Check sheet for the modelled part. Datum: model origin and axes. Units: mm. A direction names the side the tool comes from. Give positions to 0.01 mm unless a question says otherwise; leave off trailing zeros. Order: outer loops, then holes, each group sorted by start corner. A loop starts at its lowest first (then second) coordinate and runs counter-clockwise, first axis right, second up.
Item 1: Sectioned sample at B-B on x = 38.5. Record the boundary of the cut face in (y, z).
Item 2: Sectioned sample at A-A on x = 20.5. Record the boundary of the cut face in (y, z).
Item 3: Access from +Z, -Z, +X, -X, +Y, -Y to the whole of each face (thin tool, end or side, straight path). Record for faces 4 (the flat face through (63.09, -1.23, 1.48)), 5 (the flat face through (22, -4.25, 2)), 6 (the cylindrical face through (-10.248, 0.225, 1.479)), 7 (the flat face through (16, -10.25, 1)), 8 (the flat face through (54, -14.25, 9)).
Item 4: Material ranges on line 1 along Z through (x, y) = (68.5, -15.65); line 2 along Z through (x, y) = (63, -4); line 3 along Y through (x, z) = (36, 11), recorded low to high.
Item 5: Sectioned sample at C-C on y = -12.5. Record the boundary of the cut face in (x, z).
Item 6: Release check for a two-part mould opening along Z. For faces 1 (the flat face through (32, -6, 4)), 2 (the cylindrical face through (-4.25, 0.09, 1.99)), 3 (the cylindrical face through (70.837, -16.264, 9.736)) record: released by +Z, released by -Z, zero draft, split by the parting line, or undercut.
Item 7: Gauge pin test, flat ends, axial feed: P1, Ø4, axis at y = -14.5, z = 12, coming from the -X side; P2, Ø5, axis at x = 54.5, z = 7, coming from the +Y side; P3, Ø6.5, axis at x = 68.5, z = 9, coming from the -Y side. Record the tip position at first contact, or that the pin passes through.
from build123d import *

# Parameters (mm, degrees)
PAD011_DEPTH = 4
SKETCH013_W  = 42
SKETCH013_H  = 10
SKETCH013_R  = 2.45
PAD012_DEPTH = 4
FILLET005_R  = 1


with BuildPart() as part:
    # Sketch012 → Pad011 (new body)
    with BuildSketch(Plane.XY):
        with BuildLine():
            ThreePointArc((0, 10.25), (-10.25, 0), (0, -10.25))
            Line((0, -10.25), (32.5, -10.25))
            Line((32.5, -18.25), (32.5, -10.25))
            Line((32.5, -18.25), (74.5, -18.25))
            Line((74.5, -10.25), (74.5, -18.25))
            Line((74.5, -10.25), (51.355591, 8.041701))
            ThreePointArc((51.355591, 8.041701), (48.364154, 9.682199), (45, 10.25))
            Line((45, 10.25), (0, 10.25))
        make_face()
        with BuildLine():
            ThreePointArc((0, 4.25), (-4.25, 0), (0, -4.25))
            Line((0, -4.25), (45, -4.25))
            ThreePointArc((45, -4.25), (49.25, 0), (45, 4.25))
            Line((45, 4.25), (0, 4.25))
        make_face(mode=Mode.SUBTRACT)
    extrude(amount=PAD011_DEPTH)

    # Sketch013 → Pad012 (join)
    with BuildSketch(Plane(origin=(32.5, -18.25, 4), x_dir=(1, 0, 0), z_dir=(0, -1, 0))):
        with Locations((21, 5)):
            Rectangle(SKETCH013_W, SKETCH013_H)
        with Locations((6, 5)):
            Circle(SKETCH013_R, mode=Mode.SUBTRACT)
        with Locations((36, 5)):
            Circle(SKETCH013_R, mode=Mode.SUBTRACT)
    extrude(amount=-PAD012_DEPTH)

    # Fillet005
    fillet005_edges = [part.edges().sort_by_distance(p)[0] for p in [
        (0, -4.25, 2),
        (45, -4.25, 2),
        (22.5, -4.25, 0),
        (22.5, -4.25, 4),
        (70.95, -16.25, 9),
        (66.05, -18.25, 9),
        (66.05, -14.25, 9),
        (32.5, -14.25, 9),
        (16.25, -10.25, 4),
    ]]
    fillet(fillet005_edges, radius=FILLET005_R)


solid = part.part
Report:
1. outline: (-18.25, 0) - (-5.25, 0) arc R1 ccw to (-4.25, 1) - (-4.25, 3) arc R1 ccw to (-5.25, 4) - (-14.25, 4) - (-14.25, 6.55) - (-18.25, 6.55) - close; (-18.25, 11.45) - (-14.25, 11.45) - (-14.25, 14) - (-18.25, 14) - close; (4.25, 1) arc R1 ccw to (5.25, 0) - (10.25, 0) - (10.25, 3) arc R1 ccw to (9.25, 4) - (5.25, 4) arc R1 ccw to (4.25, 3) - close
2. outline: (-10.25, 0) - (-5.25, 0) arc R1 ccw to (-4.25, 1) - (-4.25, 3) arc R1 ccw to (-5.25, 4) - (-9.25, 4) arc R1 ccw to (-10.25, 3) - close; (4.25, 1) arc R1 ccw to (5.25, 0) - (10.25, 0) - (10.25, 3) arc R1 ccw to (9.25, 4) - (5.25, 4) arc R1 ccw to (4.25, 3) - close
3. face 4: +Z, -Z, +X, +Y
3. face 5: +Z, -Z
3. face 6: +Z, -Z, -X
3. face 7: +Z, -Z, -X, -Y
3. face 8: +Z, +X, -X, +Y
4. line 1: z = 0 to 6.55, 11.45 to 14
4. line 2: z = 0 to 4
4. line 3: y = -18.25 to -14.25
5. outline: (32.5, 0) - (74.5, 0) - (74.5, 4) - (32.5, 4) - close
6. face 1: released by +Z
6. face 2: zero draft
6. face 3: undercut
7. P1: stops at x = 32.5
7. P2: stops at y = -14.25
7. P3: stops at y = -18.23
